Source: CAD feature listing. Evaluate the final solid. Frame: model axes, mm. A direction names the side the tool comes from. Give positions to 0.01 mm unless a question says otherwise; leave off trailing zeros. Loops run counter-clockwise (first coordinate to the right, second up) from the corner with the lowest first, then second, coordinate; pieces in that order, holes last. Notation, with made-up numbers: M 47.25,79.5 L 86.25,79.5 A27 ccw 86.25,106.5 Z; hole C -9.75,17.5 d8. An arc over 180 degrees is marked long. Write item = value, one per line.
from build123d import *

# Parameters (mm, degrees)
SKETCH2_W           = 30
SKETCH2_H           = 130
BOSS_EXTRUDE1_DEPTH = 10
CUT_EXTRUDE3_DEPTH  = 75.64013832
FILLET3_RADIUS      = 8
FILLET3_LENGTH      = 10
FILLET4_R           = 4
SKETCH3_R           = 1.65
CUT_EXTRUDE4_DEPTH  = 75.64013841


with BuildPart() as part:
    # Sketch2 → Boss-Extrude1 (new body)
    with BuildSketch(Plane.XY):
        with Locations((-14.802371542, -2.697628458)):
            Rectangle(SKETCH2_W, SKETCH2_H)
    extrude(amount=BOSS_EXTRUDE1_DEPTH)

    # Sketch6 → Cut-Extrude3 (cut, through all)
    with BuildSketch(Plane.XY.offset(10)):
        Polygon((-29.802371542, -67.697628458), (-22.802371542, -67.697628458), (-22.802371542, -33.848814229), (-29.802371542, 0), align=None)
        Polygon((0.197628458, -67.697628458), (-6.802371542, -67.697628458), (-6.802371542, -33.848814229), (0.197628458, 0), align=None)
    extrude(amount=-CUT_EXTRUDE3_DEPTH, mode=Mode.SUBTRACT)

    # Fillet3: full round fillet: the end face becomes a half cylinder, R = half its width
    fillet3_face = Plane((-14.802371542, -67.697628458, 5), x_dir=(0, 0, 1), z_dir=(0, -1, 0))  # on the end face: x along it, z out of the body
    fillet3_slab = fillet3_face.offset(-FILLET3_RADIUS / 2) * Box(FILLET3_LENGTH, 2 * FILLET3_RADIUS, FILLET3_RADIUS, mode=Mode.PRIVATE)  # the body's end, R deep
    fillet3_round = Plane((-14.802371542, -59.697628458, 5), x_dir=(0, -1, 0), z_dir=(0, 0, 1)) * Cylinder(FILLET3_RADIUS, FILLET3_LENGTH, mode=Mode.PRIVATE)  # its axis R under the face
    add(fillet3_slab - fillet3_round, mode=Mode.SUBTRACT)

    # Fillet4
    fillet4_edges = [part.edges().sort_by_distance(p)[0] for p in [
        (0.197628458, 31.151185771, 0),
        (0.197628458, 31.151185771, 10),
        (-3.302371542, -16.924407115, 10),
        (-6.802371542, -33.848814229, 5),
        (0.197628458, 0, 5),
        (-3.302371542, -16.924407115, 0),
        (-26.302371542, -16.924407115, 10),
        (-29.802371542, 0, 5),
        (-22.802371542, -33.848814229, 5),
        (-26.302371542, -16.924407115, 0),
        (-22.802371542, -46.773221344, 10),
        (-22.802371542, -46.773221344, 0),
        (-6.802371542, -46.773221344, 10),
        (-6.802371542, -46.773221344, 0),
        (-14.802371542, -67.697628458, 0),
        (-14.802371542, -67.697628458, 10),
        (-29.802371542, 31.151185771, 10),
        (-29.802371542, 31.151185771, 0),
        (-29.802371542, 62.302371542, 5),
        (0.197628458, 62.302371542, 5),
    ]]
    fillet(fillet4_edges, radius=FILLET4_R)

    # Sketch3 → Cut-Extrude4 (cut, through all)
    with BuildSketch(Plane.XY.offset(10)):
        with Locations((-21.802371542, 42.302371542)):
            Circle(SKETCH3_R)
        with Locations((-14.802371542, 49.302371542)):
            Circle(SKETCH3_R)
        with Locations((-7.802371542, 42.302371542)):
            Circle(SKETCH3_R)
        with Locations((-14.802371542, 35.302371542)):
            Circle(SKETCH3_R)
        with Locations((-14.802371542, 42.302371542)):
            Circle(SKETCH3_R)
    extrude(amount=-CUT_EXTRUDE4_DEPTH, mode=Mode.SUBTRACT)


solid = part.part
1. Pull-direction query (X, two-part tool) for faces 6 (the cylindrical face through (-4.372, -16.462, 1.203)), 7 (the cylindrical face through (-15.2, 40.7, 5.1)), 8 (the cylindrical face through (-21.66, -46.8, 8.8)); classes: +X half, -X half, draft (parallel to the pull), parting line (faces both ways), or undercut.
Derived:
face_6 = +X half
face_7 = undercut
face_8 = -X half
2. Cut plane B-B, the plane z = 8.75. Count the separate pieces of the cut face and the enclosed holes in it, then the cut area to 3 significant figures.
Derived:
separate_pieces = 1
enclosed_holes = 5
area = 2,820 mm²
3. Material intervals for probe 1 along Y at (x, z) = (-13.5, 6.25); probe 2 along Y at (x, z) = (-15, 7.25); probe 3 along X at (y, z) = (43.5, 8.25), sorted ascending. Write a range as from..to.
Derived:
probe_1 = -67.58..34.29, 36.32..41.29, 43.32..48.29, 50.32..62.3
probe_2 = -67.49..33.66, 36.94..40.66, 43.94..47.66, 50.94..62.3
probe_3 = -29.11..-22.94, -20.67..-15.94, -13.67..-8.94, -6.67..-0.5
4. Reachability of faces 1 (the cylindrical face through (-28.66, 31.79, 8.8)), 2 (the cylindrical face through (-7.943, -47.156, 8.797)), 3 (the cylindrical face through (-7.943, -47.156, 1.203)), 4 (the cylindrical face through (-21.66, -46.8, 1.2)), 5 (the cylindrical face through (-23.112, 41.298, 5.07)) from +Z, -Z, +X, -X, +Y, -Y: full face, straight path, thin tool, end or side. Return the list, or none.
Derived:
face_1 = +Z, -X, +Y, -Y
face_2 = +Z, +X, -Y
face_3 = -Z, +X, -Y
face_4 = -Z, -X, -Y
face_5 = +Z, -Z
5. Cut plane A-A, the plane y = 5. Return the cut outline in (x, z).
Derived:
outline = M -29.8,4 A4 ccw -25.8,0 L -3.8,0 A4 ccw 0.2,4 L 0.2,6 A4 ccw -3.8,10 L -25.8,10 A4 ccw -29.8,6 Z
6. First-contact query: pin 1 Ø0.6 at (y, z) = (-44, 4.5) entering from +X; pin 2 Ø0.6 at (y, z) = (-50, 5) entering from -X; pin 3 Ø2 at (x, y) = (-14.8, 42.3) entering from +Z; pin 4 Ø1.5 at (y, z) = (-32.5, 4.5) entering from -X. Flat tips, straight axial feed; report the tip coordinate or a pass-through.
Derived:
pin_1 = -6.8
pin_2 = -22.8
pin_3 = through
pin_4 = -23.24
